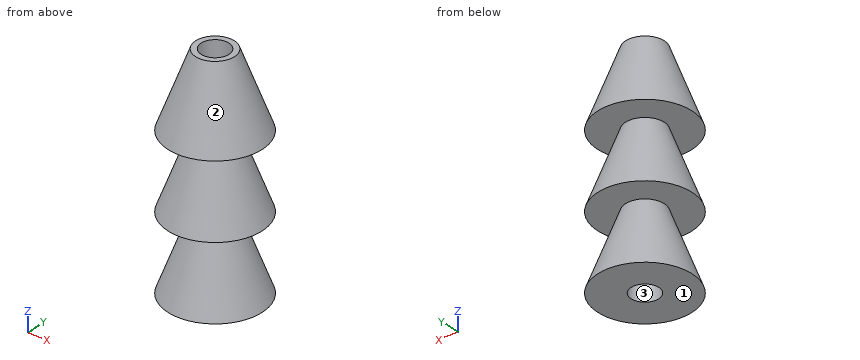
from build123d import *

# Parameters (mm, degrees)
F2_R     = 5
F3_DEPTH = 80.001


with BuildPart() as f1:
    # F0 (on Front) → F1 (revolve)
    with BuildSketch(Plane.XZ):
        Polygon((0, 40), (-7, 40), (-17, 13.333333), (-7, 13.333333), (-17, -13.333333), (-7, -13.333333), (-17, -40), (-7, -40), (0, -40), align=None)
    revolve(axis=Axis((0, 0, 0), (0, 0, -1)))

    # F2 (on face) → F3 (cut, through all)
    with BuildSketch(Plane.XY.offset(40)):
        Circle(F2_R)
    extrude(amount=-F3_DEPTH, mode=Mode.SUBTRACT)


solid = f1.part
Input: part model. Units: mm. Frame: model coordinates. Face numbers are marked on the shaded views. Give positions to 0.01 mm unless a question says otherwise; leave off trailing zeros. Order: outer loops, then holes, each group sorted by start corner. A loop starts at its lowest first (then second) coordinate and runs counter-clockwise, first axis right, second up.
Q1. Section A-A on x = 0. Output: boundary loops of the cut face in (y, z), and give its area (3 significant figures).
Checked values:
outline: (-17, -40) - (-5, -40) - (-5, 40) - (-7, 40) - (-17, 13.33) - (-7, 13.33) - (-17, -13.33) - (-7, -13.33) - close; (5, -40) - (17, -40) - (7, -13.33) - (17, -13.33) - (7, 13.33) - (17, 13.33) - (7, 40) - (5, 40) - close
area: 1,120 mm2
Q2. Draft query along Y for the marked faces 1, 2 and 3. Return one class per face: +Y half, -Y half, draft (parallel to the pull), parting line (faces both ways), or undercut.
Checked values:
face 1: draft
face 2: parting line
face 3: undercut
Q3. Section C-C on z = -19. Output: boundary loops of the cut face in (x, y) (3 decimals).
Checked values:
outline: circle Ø18.25 at (0, 0); hole circle Ø10 at (0, 0)
Q4. Ray query, probe 1 along Z at (x, y) = (11.5, -4); probe 2 along Z at (x, y) = (-9, 13.5); probe 3 along Y at (x, z) = (0, 6). Return the intervals inside material, ascending.
Checked values:
probe 1: z = -40 to -27.14, -13.33 to -0.47, 13.33 to 26.2
probe 2: z = -40 to -37.93, -13.33 to -11.27, 13.33 to 15.4
probe 3: y = -9.75 to -5, 5 to 9.75
Q5. Section D-D on x = -11. State how many separate pieces and enclosed holes the cut face has, and give its area (3 significant figures).
Checked values:
separate pieces: 3
enclosed holes: 0
area: 793 mm2
Q6. Contact query for flat-ended pins moving along their axis: pin 1 Ø12 at (y, z) = (3, 5.5) entering from +X; pin 2 Ø5 at (x, z) = (-12.5, -26.5) entering from +Y; pin 3 Ø12 at (x, z) = (0.5, 32) entering from -Y. Output: stop coordinate, or through.
Checked values:
pin 1: stops at x = 12.03
pin 2: stops at y = 6.88
pin 3: stops at y = -12.25
